Study the drawing (mm; zero at the part's minimum x, y, z) and answer. Coordinates: 2 decimals unless noted, no trailing zeros. Loops run counter-clockwise (first coordinate to the right, second up) from the corner with the lowest first, then second, coordinate; pieces in that order, holes last. Notation, with made-up numbers: (-12, 87.25) -> (11, 87.25) arc R7 ccw to (11, 96.25) -> close; hole circle Ø7 at (-34, 61.25). An arc over 180 degrees is marked (long way). Answer in a Markdown table with one row per item.
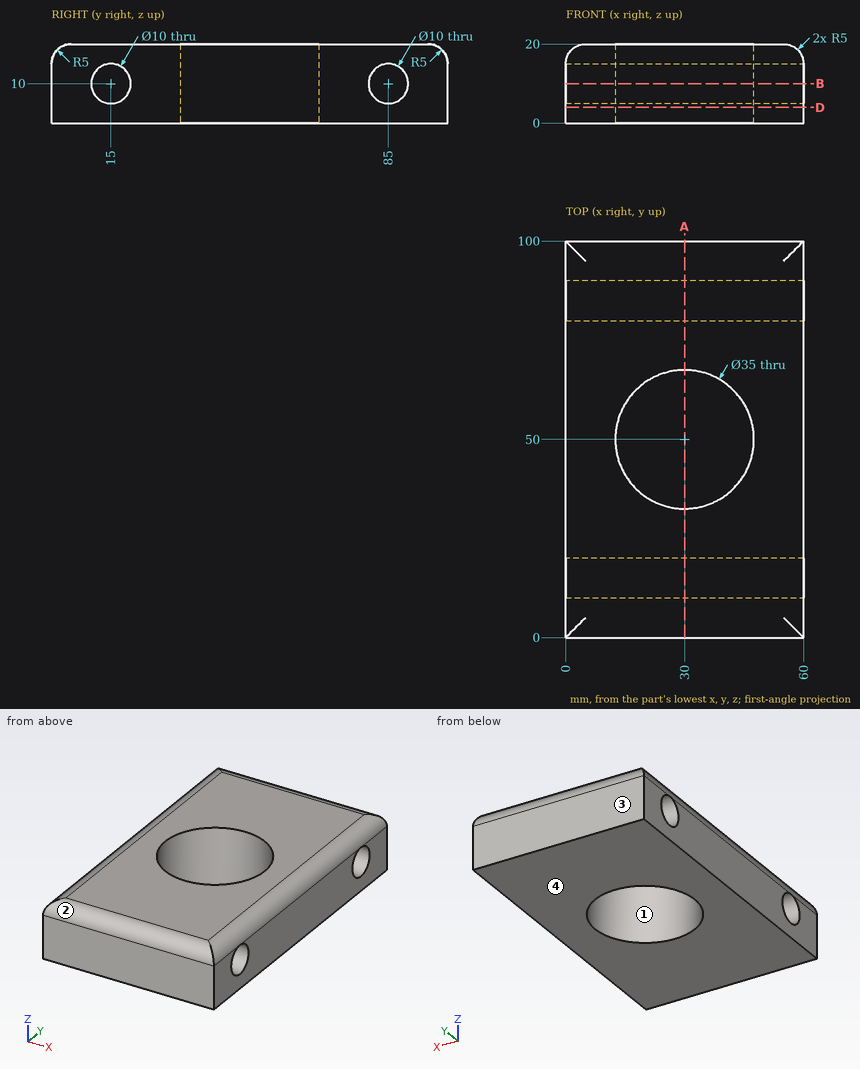
1. Find the intervals of material crossed by probe 1 along Z at (x, y) = (12.5, 15); probe 2 along Y at (x, z) = (17.5, 9); probe 3 along Y at (x, z) = (54.5, 5.5), in increasing order.
A:
| item | result |
|---|---|
| probe 1 | z = 0 to 5, 15 to 20 |
| probe 2 | y = 0 to 10.1, 19.9 to 37.75, 62.25 to 80.1, 89.9 to 100 |
| probe 3 | y = 0 to 12.82, 17.18 to 82.82, 87.18 to 100 |
2. A cutting plane is placed at A-A on x = 30. Give the vertices of the cut face in (y, z).
A:
| item | result |
|---|---|
| outline | (0, 0) -> (32.5, 0) -> (32.5, 20) -> (5, 20) arc R5 ccw to (0, 15) -> close; (67.5, 0) -> (100, 0) -> (100, 15) arc R5 ccw to (95, 20) -> (67.5, 20) -> close; hole circle Ø10 at (15, 10); hole circle Ø10 at (85, 10) |
3. A cutting plane is placed at B-B on z = 10. Give the vertices of the cut face in (x, y).
A:
| item | result |
|---|---|
| outline | (0, 0) -> (60, 0) -> (60, 10) -> (0, 10) -> close; (0, 20) -> (60, 20) -> (60, 80) -> (0, 80) -> close; (0, 90) -> (60, 90) -> (60, 100) -> (0, 100) -> close; hole circle Ø35 at (30, 50) |
4. A cutting plane is placed at D-D on z = 4. Give the vertices of the cut face in (x, y).
A:
| item | result |
|---|---|
| outline | (0, 0) -> (60, 0) -> (60, 100) -> (0, 100) -> close; hole circle Ø35 at (30, 50) |
5. The mould has two halves that part along Y. Classify the marked faces 1, 2, 3 and 4: pulls with the +Y half, pulls with the -Y half, needs draft (parallel to the pull), parting line crosses it, or undercut.
A:
| item | result |
|---|---|
| face 1 | undercut |
| face 2 | pulls with the -Y half |
| face 3 | pulls with the +Y half |
| face 4 | needs draft |
